```python
from build123d import *

# Parameters (mm, degrees)
F1_DEPTH  = 48.26
F3_DEPTH  = 8.382
F5_DEPTH  = 8.382
F6_R      = 1.8288
F7_DEPTH  = 32.8422
F8_R      = 1.8288
F9_DEPTH  = 32.8422
F11_DEPTH = 57.15
F12_W     = 2.286
F12_H     = 3.556
F13_DEPTH = 48.768
F14_R     = 2.286


with BuildPart() as f1:
    # F0 (on Top) → F1 (new body)
    with BuildSketch(Plane.XY):
        with BuildLine():
            ThreePointArc((-38.1, -38.1), (0, -50.8), (38.1, -38.1))
            Line((38.1, -38.1), (38.1, 38.1))
            ThreePointArc((38.1, 38.1), (0, 50.8), (-38.1, 38.1))
            Line((-38.1, 38.1), (-38.1, -38.1))
        make_face()
    extrude(amount=-F1_DEPTH)

    # F2 (on face) → F3 (join)
    with BuildSketch(Plane.XY):
        with BuildLine():
            Line((-34.925, 36.486888), (-34.925, -36.486888))
            ThreePointArc((-34.925, -36.486888), (0, -47.625), (34.925, -36.486888))
            Line((34.925, -36.486888), (34.925, 36.486888))
            ThreePointArc((34.925, 36.486888), (0, 47.625), (-34.925, 36.486888))
        make_face()
    extrude(amount=F3_DEPTH)

    # F4 (on face) → F5 (cut, through all)
    with BuildSketch(Plane.XY.offset(8.382)):
        with BuildLine():
            ThreePointArc((-26.67, -36.395757), (-25.275443, -31.1912), (-30.48, -29.796643))
            Line((-30.48, -29.796643), (-52.477045, -42.496643))
            ThreePointArc((-52.477045, -42.496643), (-53.871602, -47.7012), (-48.667045, -49.095757))
            Line((-48.667045, -49.095757), (-26.67, -36.395757))
        make_face()
        with BuildLine():
            Line((52.477045, -42.496643), (30.48, -29.796643))
            ThreePointArc((30.48, -29.796643), (25.275443, -31.1912), (26.67, -36.395757))
            Line((26.67, -36.395757), (48.667045, -49.095757))
            ThreePointArc((48.667045, -49.095757), (53.871602, -47.7012), (52.477045, -42.496643))
        make_face()
        with BuildLine():
            Line((-52.477045, 42.496643), (-30.48, 29.796643))
            ThreePointArc((-30.48, 29.796643), (-25.275443, 31.1912), (-26.67, 36.395757))
            Line((-26.67, 36.395757), (-48.667045, 49.095757))
            ThreePointArc((-48.667045, 49.095757), (-53.871602, 47.7012), (-52.477045, 42.496643))
        make_face()
        with BuildLine():
            ThreePointArc((26.67, 36.395757), (25.275443, 31.1912), (30.48, 29.796643))
            Line((30.48, 29.796643), (52.477045, 42.496643))
            ThreePointArc((52.477045, 42.496643), (53.871602, 47.7012), (48.667045, 49.095757))
            Line((48.667045, 49.095757), (26.67, 36.395757))
        make_face()
    extrude(amount=-F5_DEPTH, mode=Mode.SUBTRACT)

    # F6 (on face) → F7 (cut)
    with BuildSketch(Plane.XY):
        with Locations((-28.575, 33.0962)):
            Circle(F6_R)
        with Locations((28.575, 33.0962)):
            Circle(F6_R)
        with Locations((28.575, -33.0962)):
            Circle(F6_R)
        with Locations((-28.575, -33.0962)):
            Circle(F6_R)
    extrude(amount=-F7_DEPTH, mode=Mode.SUBTRACT)

    # F8 (on face) → F9 (cut)
    with BuildSketch(Plane.XY):
        with Locations((-28.575, 33.0962)):
            Circle(F8_R)
        with Locations((28.575, 33.0962)):
            Circle(F8_R)
        with Locations((28.575, -33.0962)):
            Circle(F8_R)
        with Locations((-28.575, -33.0962)):
            Circle(F8_R)
    extrude(amount=-F9_DEPTH, mode=Mode.SUBTRACT)

    # F10 (on Top) → F11 (join)
    with BuildSketch(Plane.XY):
        with BuildLine():
            ThreePointArc((-12.7, 6.35), (0, -6.35), (12.7, 6.35))
            Line((12.7, 6.35), (12.7, 31.75))
            ThreePointArc((12.7, 31.75), (0, 44.45), (-12.7, 31.75))
            Line((-12.7, 31.75), (-12.7, 6.35))
        make_face()
    extrude(amount=F11_DEPTH)

    # F12 (on face) → F13 (join, through all)
    with BuildSketch(Plane.XY.offset(8.382)):
        with Locations((-13.843, 11.684)):
            Rectangle(F12_W, F12_H)
    extrude(amount=F13_DEPTH)

    # F14
    f14_edges = [f1.edges().sort_by_distance(p)[0] for p in [
        (12.7, 19.05, 57.15),
    ]]
    fillet(f14_edges, radius=F14_R)


solid = f1.part
```
The model under review builds one solid part; all positions refer to its coordinate system, in mm. A direction names the side the tool comes from. Round coordinates to 2 decimals unless told otherwise and drop trailing zeros. Loops run counter-clockwise (first coordinate to the right, second up) from the corner with the lowest first, then second, coordinate; pieces in that order, holes last.
Item 1: For line 1 (Z direction, x = 13, y = -32); line 2 (X direction, y = 29.5, z = 20); line 3 (Y direction, x = -1, z = 20.5), list the stretches that pass through material, from the lowest coordinate up.
Determined:
line 1: z = -48.26 to 8.38
line 2: x = -12.7 to 12.7
line 3: y = -6.31 to 44.41
Item 2: Take a section at B-B (y = -21). Write out the cut boundary in (x, z) (3 decimals).
Determined:
outline: (-38.1, -48.26) - (38.1, -48.26) - (38.1, 0) - (34.925, 0) - (34.925, 8.382) - (-34.925, 8.382) - (-34.925, 0) - (-38.1, 0) - close
Item 3: Clearance check with flat-ended pins moving along their axes: pin 1 Ø1.5 at (x, y) = (9.5, -12) entering from +Z; pin 2 Ø3 at (x, y) = (29, -34) entering from +Z; pin 3 Ø3.5 at (x, y) = (28.58, -33.1) entering from +Z. State where each tip first meets the part, or that it passes through.
Determined:
pin 1: stops at z = 8.38
pin 2: stops at z = 0
pin 3: stops at z = -32.84
Item 4: For faces 4 (the face through (-0.279, -6.347, 31.298)), 5 (the face through (-28.93, -37.7, 4.25)), 6 (the face through (-25.318, 31.119, 4.25)), 7 (the face through (34.925, 0, 4)), list the 3-axis set-ups (+Z, -Z, +X, -X, +Y, -Y) from which the entire face can be reached by the end or side of a thin tool; tool diameter is ignored.
Determined:
face 4: +Z, -Y
face 5: +Z, -X
face 6: +Z
face 7: +Z, +X, +Y, -Y
Item 5: Mouldability with a two-part tool opening along Y and no side actions: class faces 1 (the face through (-0.458, -47.623, 4.132)), 2 (the face through (-12.7, 23, 31)), 3 (the face through (-29, -33, -32.842)) as released by +Y, released by -Y, zero draft, split by the parting line, or undercut.
Determined:
face 1: released by -Y
face 2: zero draft
face 3: undercut
Item 6: Take a section at C-C (z = 21). Write out the cut boundary in (x, y).
Determined:
outline: (-14.99, 9.91) - (-12.7, 9.91) - (-12.7, 6.35) arc R12.7 ccw to (12.7, 6.35) - (12.7, 31.75) arc R12.7 ccw to (-12.7, 31.75) - (-12.7, 13.46) - (-14.99, 13.46) - close
Item 7: Take a section at A-A (x = 0). Write out the cut boundary in (y, z) (3 decimals).
Determined:
outline: (-50.8, -48.26) - (50.8, -48.26) - (50.8, 0) - (47.625, 0) - (47.625, 8.382) - (44.45, 8.382) - (44.45, 54.864) arc R2.286 ccw to (42.164, 57.15) - (-4.064, 57.15) arc R2.286 ccw to (-6.35, 54.864) - (-6.35, 8.382) - (-47.625, 8.382) - (-47.625, 0) - (-50.8, 0) - close
Item 8: Take a section at D-D (z = -26.5). Write out the cut boundary in (x, y) (3 decimals), then the cut area to 3 significant figures.
Determined:
outline: (-38.1, -38.1) arc R63.5 ccw to (38.1, -38.1) - (38.1, 38.1) arc R63.5 ccw to (-38.1, 38.1) - close; hole circle Ø3.658 at (-28.575, -33.096); hole circle Ø3.658 at (-28.575, 33.096); hole circle Ø3.658 at (28.575, -33.096); hole circle Ø3.658 at (28.575, 33.096)
area: 7,080 mm2
